Autodesk Inventor part; units mm, degrees
ref_plane "YZ Plane" through (0, 0, 0) normal (1, 0, 0) x (0, 1, 0)
ref_plane "XZ Plane" through (0, 0, 0) normal (0, 1, 0) x (-1, 0, 0)
ref_plane "XY Plane" through (0, 0, 0) normal (0, 0, 1) x (1, 0, 0)
sketch "main" plane through (0, 0, 0) normal (0, 0, 1) x (1, 0, 0)
  circle A0 centre (18.656, 25.5497) radius 2.1844
  circle A1 centre (-6.744, 25.5497) radius 2.1844
  line L0 (-6.744, 16.0247) -> (-6.744, -15.7253)
  line L1 (-0.394, -30.5843) -> (25.006, 17.6122)
  arc A2 (-6.744, 16.0247) -> (-9.919, 19.1997) centre (-9.919, 16.0247) ccw
  line L2 (-19.444, 19.1997) -> (-9.919, 19.1997)
  circle A3 centre (-19.444, 25.5497) radius 2.1844
  arc A4 (-19.444, 31.8997) -> (-19.444, 19.1997) centre (-19.444, 25.5497) ccw
  line L3 (25.006, 25.5497) -> (25.006, 17.6122)
  line L4 (18.656, 31.8997) -> (-19.444, 31.8997)
  arc A5 (25.006, 25.5497) -> (18.656, 31.8997) centre (18.656, 25.5497) ccw
  arc A6 (-9.919, -18.9003) -> (-6.744, -15.7253) centre (-9.919, -15.7253) ccw
  line L5 (-19.444, -18.9003) -> (-9.919, -18.9003)
  circle A7 centre (-6.744, -25.2503) radius 2.1844
  line L6 (-0.394, -30.5843) -> (-1.41, -31.6003)
  circle A8 centre (-19.444, -25.2503) radius 2.1844
  arc A9 (-19.444, -18.9003) -> (-19.444, -31.6003) centre (-19.444, -25.2503) ccw
  line L7 (-1.41, -31.6003) -> (-19.444, -31.6003)
  circle A10 centre (9.131, 6.4997) radius 2.0955
  point P0 (-4.4485, 2.2347)
  dimension "d0" = 3.175
  dimension "d3" = 4.191
sketch "Sketch1" plane through (0, 0, 0) normal (0, 1, 0) x (-1, 0, 0)
  circle A0 centre (38.1, 0) radius 2.1844
  circle A1 centre (12.7, 0) radius 2.1844
  line L0 (12.7, -9.525) -> (12.7, -41.275)
  line L1 (19.05, -56.134) -> (44.45, -7.9375)
  arc A2 (12.7, -9.525) -> (9.525, -6.35) centre (9.525, -9.525) ccw
  line L2 (0, -6.35) -> (9.525, -6.35)
  circle A3 centre (0, 0) radius 2.1844
  arc A4 (0, 6.35) -> (0, -6.35) centre (0, 0) ccw
  line L3 (44.45, 0) -> (44.45, -7.9375)
  line L4 (38.1, 6.35) -> (0, 6.35)
  arc A5 (44.45, 0) -> (38.1, 6.35) centre (38.1, 0) ccw
  arc A6 (9.525, -44.45) -> (12.7, -41.275) centre (9.525, -41.275) ccw
  line L5 (0, -44.45) -> (9.525, -44.45)
  circle A7 centre (12.7, -50.8) radius 2.1844
  line L6 (19.05, -56.134) -> (18.034, -57.15)
  circle A8 centre (0, -50.8) radius 2.1844
  arc A9 (0, -44.45) -> (0, -57.15) centre (0, -50.8) ccw
  line L7 (18.034, -57.15) -> (0, -57.15)
  circle A10 centre (28.575, -19.05) radius 2.0955
extrude "Extrusion1" add sketch "Sketch1" along normal blind 1.5875
properties part number "gusset" material "Acetal Resin, White"
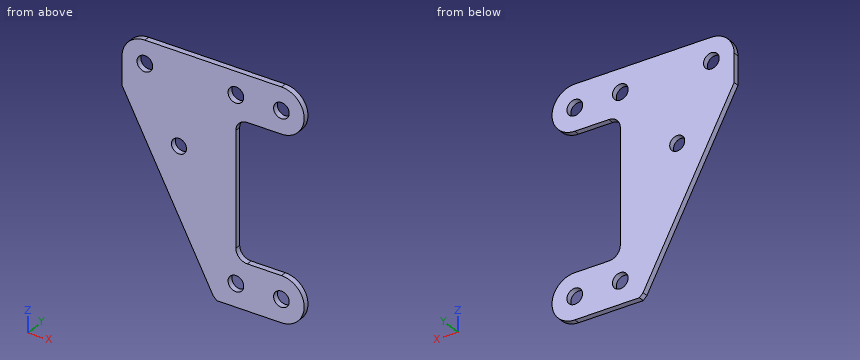
The model under review builds one solid part; all positions refer to its coordinate system, in mm. Give positions to 0.01 mm unless a question says otherwise; leave off trailing zeros. Loops run counter-clockwise (first coordinate to the right, second up) from the corner with the lowest first, then second, coordinate; pieces in that order, holes last. Notation, with made-up numbers: (-39.5, 60.5) -> (-21.5, 60.5) arc R20 cw to (-21.5, 87.5) -> close; hole circle Ø6 at (-19, 67.5). An arc over 180 degrees is marked (long way). Use CSV: the item, a comma, the result in double quotes.
1. Consider section D-D, the plane z = -19.05. Write out the cut boundary in (x, y).
Result:
outline,"(-38.59, 0) -> (-30.67, 0) -> (-30.67, 1.59) -> (-38.59, 1.59) -> close; (-26.48, 0) -> (-12.7, 0) -> (-12.7, 1.59) -> (-26.48, 1.59) -> close"
2. For P1, Ø0.5, axis at y = 1, z = -30, coming from the +X side; P2, Ø4, axis at x = 0, z = 0, coming from the -Y side, all flat-tipped, find the tip position at first contact; note any pin that passes through.
Result:
P1,"stops at x = -12.7"
P2,"passes through"
3. Consider section A-A, the plane z = -50.8. Write out the cut boundary in (x, y), then the cut area to 3 significant figures.
Result:
outline,"(-21.86, 0) -> (-14.88, 0) -> (-14.88, 1.59) -> (-21.86, 1.59) -> close; (-10.52, 0) -> (-2.18, 0) -> (-2.18, 1.59) -> (-10.52, 1.59) -> close; (2.18, 0) -> (6.35, 0) -> (6.35, 1.59) -> (2.18, 1.59) -> close"
area,"30.9 mm²"
4. Consider section B-B, the plane x = -8.5. Write out the cut boundary in (y, z), then the cut area to 3 significant figures.
Result:
outline,"(0, -57.15) -> (1.59, -57.15) -> (1.59, -44.45) -> (0, -44.45) -> close; (0, -6.35) -> (1.59, -6.35) -> (1.59, 6.35) -> (0, 6.35) -> close"
area,"40.3 mm²"
5. Consider section C-C, the plane y = 0.95. Count the separate pieces of the cut face and the enclosed holes in it, then the cut area to 3 significant figures.
Result:
separate pieces,"1"
enclosed holes,"6"
area,"1,730 mm²"
6. To check wall thickness, follow probe 1 along Z at (x, y) = (0, 0.45); probe 2 along Z at (x, y) = (1.5, 0.3); probe 3 along X at (y, z) = (0.5, -49). State the ranges of each line that lie inside material, in increasing order. Write a range as from..to.
Result:
probe 1,"z = -57.15..-52.98, -48.62..-44.45, -6.35..-2.18, 2.18..6.35"
probe 2,"z = -56.97..-52.39, -49.21..-44.63, -6.17..-1.59, 1.59..6.17"
probe 3,"x = -22.81..-13.94, -11.46..-1.24, 1.24..6.09"
